Check sheet for the modelled part. Datum: model origin and axes. Units: mm. Round coordinates to 2 decimals unless told otherwise and drop trailing zeros. Answer in a Markdown table with one row per item. Add a question column.
1. Sectioned sample at A-A, the plane y = 0.15. Count the separate pieces of the cut face and the enclosed holes in it, then the cut area to 3 significant figures.
2. Material ranges on L1, parallel to X at y = 0.1, z = 42; L2, parallel to X at y = 0.15, z = -30.5; L3, parallel to Z at x = -36.5, y = -0.25, recorded low to high. Write a range as from..to.
3. Depth check by flat-ended pin: P1, Ø1.5, axis at x = 11, y = -0.5, coming from the -Z side; P2, Ø2.5, axis at x = -50.14, z = 42.42, coming from the -Y side; P3, Ø1.6, axis at x = 29, y = -0.5, coming from the +Z side; P4, Ø1, axis at x = -64, y = 0.5, coming from the -Z side. Enter the tip coordinate at first touch or a pass-through.
```python
from build123d import *

# Parameters (mm, degrees)
BOSS_EXTRUDE4_DEPTH  = 1.5875
M3_CLEARANCE_HOLE3_D = 3
M3_CLEARANCE_HOLE1_D = 3.1
M3_CLEARANCE_HOLE4_D = 2.95
M3_CLEARANCE_HOLE2_D = 3.1
BOSS_EXTRUDE6_DEPTH  = 3.175
FILLET1_R            = 2
FILLET3_R            = 1
FILLET6_R            = 0.5
SKETCH28_W           = 54
SKETCH28_H           = 45
CUT_EXTRUDE4_DEPTH   = 10
CUT_EXTRUDE5_DEPTH   = 10
SKETCH31_R           = 1.5
CUT_EXTRUDE7_DEPTH   = 10


with BuildPart() as part:
    # Sketch1 → Boss-Extrude4 (new, symmetric)
    with BuildSketch(Plane(origin=(0, 0, 0), x_dir=(1, 0, 0), z_dir=(0, 1, 0))):
        with BuildLine():
            Line((-62.799553621, 32.496136604), (-73.969425011, 32.691107434))
            Line((-73.969425011, 32.691107434), (-77.053684287, 35.88495141))
            ThreePointArc((-77.053684287, 35.88495141), (-84.36642289, 10.358894189), (-83.446216027, -16.178041625))
            Line((-83.446216027, -16.178041625), (-79.680911643, -13.825218315))
            Line((-79.680911643, -13.825218315), (-69.484649137, -16.179210996))
            Line((-69.484649137, -16.179210996), (-43.894490772, -57.132025032))
            Line((-43.894490772, -57.132025032), (-43.894490772, -64.826600275))
            Line((-43.894490772, -64.826600275), (-43.094490772, -64.826600275))
            Line((-43.094490772, -64.826600275), (-34, -64.826600275))
            Line((-34, -64.826600275), (-34, -62.55))
            Line((-34, -62.55), (-34, -61.55))
            Line((-34, -61.55), (-20, -61.55))
            Line((-20, -61.55), (-19.859459165, -62.55))
            Line((-19.859459165, -62.55), (19.859459165, -62.55))
            Line((19.859459165, -62.55), (20, -61.55))
            Line((20, -61.55), (34, -61.55))
            Line((34, -61.55), (34, -62.55))
            Line((34, -62.55), (34, -64.826600275))
            Line((34, -64.826600275), (43.094490772, -64.826600275))
            Line((43.094490772, -64.826600275), (43.894490772, -64.826600275))
            Line((43.894490772, -64.826600275), (43.894490772, -57.132025032))
            Line((43.894490772, -57.132025032), (69.484649137, -16.179210996))
            Line((69.484649137, -16.179210996), (79.680911643, -13.825218315))
            Line((79.680911643, -13.825218315), (83.446216027, -16.178041625))
            ThreePointArc((83.446216027, -16.178041625), (84.610662337, -8.126242604), (85, 0))
            ThreePointArc((85, 0), (82.98964744, 18.377116688), (77.053684287, 35.88495141))
            Line((77.053684287, 35.88495141), (73.969425011, 32.691107434))
            Line((73.969425011, 32.691107434), (62.799553621, 32.496136604))
            Line((62.799553621, 32.496136604), (30.284668021, 63.895396642))
            Line((30.284668021, 63.895396642), (30.089697191, 75.065268032))
            Line((30.089697191, 75.065268032), (33.173956467, 78.259112008))
            ThreePointArc((33.173956467, 78.259112008), (0, 85), (-33.173956467, 78.259112008))
            Line((-33.173956467, 78.259112008), (-30.089697191, 75.065268032))
            Line((-30.089697191, 75.065268032), (-30.284668021, 63.895396642))
            Line((-30.284668021, 63.895396642), (-62.799553621, 32.496136604))
        make_face()
    extrude(amount=BOSS_EXTRUDE4_DEPTH, both=True)

    # M3 Clearance Hole3 (through all)
    with Locations(Plane(origin=(0, -1.5875, 0), x_dir=(-1, 0, 0), z_dir=(0, -1, 0))):
        with Locations((36.5, -50), (36.5, -38), (-36.5, -50), (-36.5, -38)):
            Hole(M3_CLEARANCE_HOLE3_D / 2)

    # M3 Clearance Hole1 (through all)
    with Locations(Plane(origin=(0, 1.5875, 0), x_dir=(1, 0, 0), z_dir=(0, 1, 0))):
        with Locations((-78.542321426, -8.49139241), (78.542321426, -8.49139241), (74.155025063, 27.240269049), (-74.155025063, 27.240269049)):
            Hole(M3_CLEARANCE_HOLE1_D / 2)

    # M3 Clearance Hole4 (through all)
    with Locations(Plane(origin=(0, -1.5875, 0), x_dir=(-1, 0, 0), z_dir=(0, -1, 0))):
        with Locations((-67.099301622, -15.278865202), (-50.141885166, -42.416404279), (-61.062544382, 30.698137949), (-38.043670771, 52.927205804), (50.141885166, -42.416404279), (67.099301622, -15.278865202), (38.043670771, 52.927205804), (61.062544382, 30.698137949)):
            Hole(M3_CLEARANCE_HOLE4_D / 2)

    # M3 Clearance Hole2 (through all)
    with Locations(Plane(origin=(0, 1.5875, 0), x_dir=(1, 0, 0), z_dir=(0, 1, 0))):
        with Locations((27, 76.497766718), (-27, 76.497766718)):
            Hole(M3_CLEARANCE_HOLE2_D / 2)

    # Sketch22 → Boss-Extrude6 (add)
    with BuildSketch(Plane(origin=(0, 1.5875, 0), x_dir=(1, 0, 0), z_dir=(0, 1, 0))):
        Polygon((65.061950694, 32.535626892), (30.245177733, 66.157793715), (30.284668021, 63.895396642), (62.799553621, 32.496136604), align=None)
        Polygon((-30.284668021, 63.895396642), (-30.245177733, 66.157793715), (-65.061950694, 32.535626892), (-62.799553621, 32.496136604), align=None)
        Polygon((43.894490772, -60.151352895), (71.689396914, -15.670204865), (69.484649137, -16.179210996), (43.894490772, -57.132025032), align=None)
        Polygon((-69.484649137, -16.179210996), (-71.689396914, -15.670204865), (-43.894490772, -60.151352895), (-43.894490772, -57.132025032), align=None)
    extrude(amount=-BOSS_EXTRUDE6_DEPTH)

    # Fillet1
    fillet1_edges = [part.edges().sort_by_distance(p)[0] for p in [
        (-30.245177733, 0.79375, -66.157793715),
        (-65.061950694, 0.79375, -32.535626892),
        (-71.689396914, 0.79375, 15.670204865),
        (-43.894490772, 0.79375, 60.151352895),
        (43.894490772, -0.79375, 60.151352895),
        (71.689396914, -0.79375, 15.670204865),
        (65.061950694, 0.79375, -32.535626892),
        (30.245177733, -0.79375, -66.157793715),
        (30.089697191, -0.79375, -75.065268032),
        (73.969425011, -0.79375, -32.691107434),
        (79.680911643, -0.79375, 13.825218315),
        (-79.680911643, -0.79375, 13.825218315),
        (-73.969425011, -0.79375, -32.691107434),
        (-30.089697191, -0.79375, -75.065268032),
    ]]
    fillet(fillet1_edges, radius=FILLET1_R)

    # Fillet3
    fillet3_edges = [part.edges().sort_by_distance(p)[0] for p in [
        (33.173956467, -0.79375, -78.259112008),
        (77.053684287, 0.79375, -35.88495141),
        (83.446216027, -0.79375, 16.178041625),
        (43.894490772, -0.79375, 64.826600275),
        (34, 0.79375, 64.826600275),
        (34, -0.79375, 61.55),
        (-34, -0.79375, 61.55),
        (-34, 0.79375, 64.826600275),
        (-43.894490772, -0.79375, 64.826600275),
        (-83.446216027, -0.79375, 16.178041625),
        (-77.053684287, -0.79375, -35.88495141),
        (-33.173956467, -0.79375, -78.259112008),
    ]]
    fillet(fillet3_edges, radius=FILLET3_R - 0.0001)  # a hair under: the kernel refuses the full size

    # Fillet6
    fillet6_edges = [part.edges().sort_by_distance(p)[0] for p in [
        (20, -0.79375, 61.55),
        (19.859459165, -0.79375, 62.55),
        (-19.859459165, 0.79375, 62.55),
        (-20, 0.79375, 61.55),
    ]]
    fillet(fillet6_edges, radius=FILLET6_R)

    # Sketch28 → Cut-Extrude4 (cut)
    with BuildSketch(Plane(origin=(0, 1.5875, 0), x_dir=(1, 0, 0), z_dir=(0, 1, 0))):
        with Locations((0, -40.05)):
            Rectangle(SKETCH28_W, SKETCH28_H)
    extrude(amount=-CUT_EXTRUDE4_DEPTH, mode=Mode.SUBTRACT)

    # Sketch29 → Cut-Extrude5 (cut)
    with BuildSketch(Plane(origin=(0, 1.5875, 0), x_dir=(1, 0, 0), z_dir=(0, 1, 0))):
        with BuildLine():
            ThreePointArc((-31.75, -56.55), (-30.25, -58.05), (-28.75, -56.55))
            Line((-28.75, -56.55), (-30.25, -56.55))
            Line((-30.25, -56.55), (-31.75, -56.55))
        make_face()
        with BuildLine():
            Line((-30.25, -56.55), (-28.75, -56.55))
            ThreePointArc((-28.75, -56.55), (-30.25, -55.05), (-31.75, -56.55))
            Line((-31.75, -56.55), (-30.25, -56.55))
        make_face()
        with BuildLine():
            ThreePointArc((28.75, -56.55), (30.25, -58.05), (31.75, -56.55))
            ThreePointArc((31.75, -56.55), (30.25, -55.05), (28.75, -56.55))
        make_face()
    extrude(amount=-CUT_EXTRUDE5_DEPTH, mode=Mode.SUBTRACT)

    # Sketch31 → Cut-Extrude7 (cut)
    with BuildSketch(Plane(origin=(0, 1.5875, 0), x_dir=(1, 0, 0), z_dir=(0, 1, 0))):
        with Locations(Location((-26, -14.55, 0), (0, 0, 270))):
            Circle(SKETCH31_R)
        with Locations(Location((26, -14.55, 0), (0, 0, 270))):
            Circle(SKETCH31_R)
    extrude(amount=-CUT_EXTRUDE7_DEPTH, mode=Mode.SUBTRACT)


solid = part.part
```
Answer key:
| question | item | result |
|---|---|---|
| 1 | separate pieces | 1 |
| 1 | enclosed holes | 22 |
| 1 | area | 15,100 mm² |
| 2 | L1 | x = -55.24..-51.56, -48.73..-27, 27..48.73, 51.56..55.24 |
| 2 | L2 | x = -79.34..-62.52, -59.6..59.6, 62.52..79.34 |
| 2 | L3 | z = -60.12..36.5, 39.5..48.5, 51.5..64.83 |
| 3 | P1 | stops at z = -84.38 |
| 3 | P2 | passes through |
| 3 | P3 | stops at z = 61.55 |
| 3 | P4 | stops at z = -34.04 |
